```python
from build123d import *

# Parameters (mm, degrees)
BOSS_EXTRUDE1_DEPTH = 65
SKETCH2_W           = 5.2
SKETCH2_H           = 2.4
CUT_EXTRUDE1_DEPTH  = 6
LPATTERN1_COUNT     = 3
LPATTERN1_PITCH     = 20
SKETCH3_W           = 12
SKETCH3_H           = 2.4
CUT_EXTRUDE2_DEPTH  = 6
FILLET1_R           = 4
FILLET2_R           = 4
SKETCH5_W           = 13.2
SKETCH5_H           = 3.1
CUT_EXTRUDE3_DEPTH  = 10
LPATTERN2_COUNT     = 2
LPATTERN2_PITCH     = 20


with BuildPart() as part:
    # Sketch1 → Boss-Extrude1 (new body)
    with BuildSketch(Plane.XY):
        Polygon((0, 0), (3.2, 0), (4.2, 0.663324958), (4.2, 3.063324958), (-1, 3.063324958), (-1, 0.663324958), align=None)
    extrude(amount=BOSS_EXTRUDE1_DEPTH)

    # Sketch2 → Cut-Extrude1 (cut)
    with BuildSketch(Plane.ZY.offset(1)):
        with Locations((3.8, 1.863324958)):
            Rectangle(SKETCH2_W, SKETCH2_H)
    cut_extrude1 = extrude(amount=-CUT_EXTRUDE1_DEPTH, mode=Mode.SUBTRACT)

    # LPattern1: Cut-Extrude1 ×3
    with Locations(*[(0, 0, i * LPATTERN1_PITCH) for i in range(1, LPATTERN1_COUNT)]):
        add(cut_extrude1, mode=Mode.SUBTRACT)

    # Sketch3 → Cut-Extrude2 (cut)
    with BuildSketch(Plane.ZY.offset(1)):
        with Locations((57.4, 1.863324958)):
            Rectangle(SKETCH3_W, SKETCH3_H)
    extrude(amount=-CUT_EXTRUDE2_DEPTH, mode=Mode.SUBTRACT)

    # Fillet1
    # the kernel refuses this fillet: 4 mm, written as the material it adds along each edge
    with BuildSketch(Plane(origin=(-1, 0.663324958, 51.4), x_dir=(0, 0, 1), z_dir=(1, 0, 0))) as fillet1_piece_1_section:
        with BuildLine():
            CenterArc((3.666060556, -4), FILLET1_R, 90, 66.421821522)
            Line((0, -2.4), (-0.073321211, -2.368))
            ThreePointArc((-0.073321211, -2.368), (-0.08, -1.2), (-0.08, 0))
            Line((-0.08, 0), (0, 0.08))
            Line((0, 0.08), (3.666060556, 0.08))
            Line((3.666060556, 0.08), (3.666060556, 0))
        make_face()
    fillet1_piece_1 = extrude(amount=5.2, mode=Mode.PRIVATE)
    fillet1_piece_1 = split(fillet1_piece_1, bisect_by=Plane(origin=(0.518931728, -0.344220367, 52.290586237), z_dir=(0.5527707983925672, 0.833333333333333, 0)), keep=Keep.TOP, mode=Mode.PRIVATE)
    fillet1_piece_1 = split(fillet1_piece_1, bisect_by=Plane(origin=(2.681068272, -0.344220367, 52.290586237), z_dir=(-0.5527707983925666, 0.8333333333333335, 0)), keep=Keep.TOP, mode=Mode.PRIVATE)
    add(fillet1_piece_1)

    # Fillet2
    # the kernel refuses this fillet: 4 mm, written as the material it adds along each edge
    with BuildSketch(Plane(origin=(-1, 0.663324958, 63.4), x_dir=(0, 1, 0), z_dir=(1, 0, 0))) as fillet2_piece_1_section:
        with BuildLine():
            CenterArc((4, -3.666060556), FILLET2_R, 113.578178478, 66.421821522)
            Line((0, -3.666060556), (-0.08, -3.666060556))
            Line((-0.08, -3.666060556), (-0.08, 0))
            Line((-0.08, 0), (0, 0.08))
            ThreePointArc((0, 0.08), (1.2, 0.08), (2.368, 0.073321211))
            Line((2.368, 0.073321211), (2.4, 0))
        make_face()
    fillet2_piece_1 = extrude(amount=5.2, mode=Mode.PRIVATE)
    fillet2_piece_1 = split(fillet2_piece_1, bisect_by=Plane(origin=(2.681068272, -0.344220367, 62.509413763), z_dir=(-0.5527707983925666, 0.8333333333333335, 0)), keep=Keep.TOP, mode=Mode.PRIVATE)
    fillet2_piece_1 = split(fillet2_piece_1, bisect_by=Plane(origin=(0.518931728, -0.344220367, 62.509413763), z_dir=(0.5527707983925672, 0.833333333333333, 0)), keep=Keep.TOP, mode=Mode.PRIVATE)
    add(fillet2_piece_1)

    # Sketch5 → Cut-Extrude3 (cut)
    with BuildSketch(Plane.ZY.offset(1)):
        with Locations((13.8, 1.113324958)):
            Rectangle(SKETCH5_W, SKETCH5_H)
    cut_extrude3 = extrude(amount=-CUT_EXTRUDE3_DEPTH, mode=Mode.SUBTRACT)

    # LPattern2: Cut-Extrude3 ×2
    with Locations(*[(0, 0, i * LPATTERN2_PITCH) for i in range(1, LPATTERN2_COUNT)]):
        add(cut_extrude3, mode=Mode.SUBTRACT)


solid = part.part
```
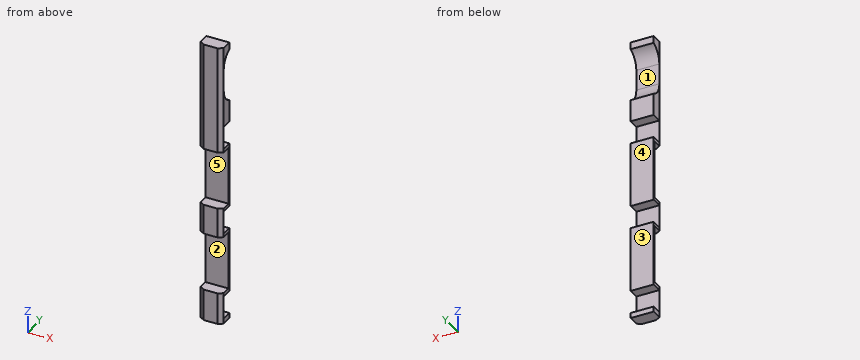
Can you work these out from the model? Positions are in its coordinate system, mm. Face numbers are marked on the shaded views. A direction names the side the tool comes from. Give positions to 0.01 mm unless a question says otherwise; leave off trailing zeros. Loops run counter-clockwise (first coordinate to the right, second up) from the corner with the lowest first, then second, coordinate; pieces in that order, holes last. Notation, with made-up numbers: M 88,-8.5 L 138,-8.5 A4 cw 138,-4.5 Z; hole C 21,-11 d9. An arc over 180 degrees is marked long. Use CSV: the item, a comma, the result in double quotes. Start each with the question number.
1. Imagine slicing it at C-C, the plane z = 50. Write out the boundary of the cut face in (x, y), plus the area to 3 significant figures.
2. If we mould it in two halves opening along Z, with no side actions, what happens to the marked faces 4 and 5? For each: released by +Z, released by -Z, zero draft, split by the parting line, or undercut.
3. If I drill on L1, parallel to Z at x = 2.45, y = 0.6; L2, parallel to Z at x = 3.95, y = 2.7; L3, parallel to Y at x = 3.7, z = 36.5, over which ranges is the centre line in solid material (lowest first)?
4. Imagine slicing it at A-A, the plane y = 1.3. Write out the boundary of the cut face in (x, z).
5. On a 3-axis mill with a long thin cutter (end or side, diameter ignored), from which of +Z, -Z, +X, -X, +Y, -Y can I reach the whole of each face in a straight line? I mean the marked faces 1, 2 and 3. Say none if no direction works.
6. For P1, Ø2.5, axis at x = 1, z = 23.5, coming from the +Y side; P2, Ø1, axis at x = 2, z = 28, coming from the -Y side, each with a flat end and sliding along its axis, tell me the tip position at first contact or that it passes through.
7. Imagine slicing it at D-D, the plane z = 8. Write out the boundary of the cut face in (x, y).
8. Imagine slicing it at B-B, the plane x = 1.5. Write out the boundary of the cut face in (y, z).
Response values:
1,outline,"M -1,0.66 L 0,0 L 3.2,0 L 4.2,0.66 L 4.2,3.06 L -1,3.06 Z"
1,area,"15.3 mm^2"
2,face 4,"zero draft"
2,face 5,"undercut"
3,L1,"0 to 7.2, 20.4 to 27.2, 40.4 to 65"
3,L2,"0 to 1.2, 6.4 to 21.2, 26.4 to 41.2, 46.4 to 51.58, 63.22 to 65"
3,L3,"2.66 to 3.06"
4,outline,"M -1,0 L 4.2,0 L 4.2,1.2 L -1,1.2 Z; M -1,6.4 L 4.2,6.4 L 4.2,7.2 L -1,7.2 Z; M -1,20.4 L 4.2,20.4 L 4.2,21.2 L -1,21.2 Z; M -1,26.4 L 4.2,26.4 L 4.2,27.2 L -1,27.2 Z; M -1,40.4 L 4.2,40.4 L 4.2,41.2 L -1,41.2 Z; M -1,46.4 L 4.2,46.4 L 4.2,52.9 L -1,52.9 Z; M -1,61.9 L 4.2,61.9 L 4.2,65 L -1,65 Z"
5,face 1,"+X, -X, +Y"
5,face 2,"+X, -X, -Y"
5,face 3,"+Z, -Z, +X, -X, +Y"
6,P1,"y = 0.66"
6,P2,"y = 2.66"
7,outline,"M -1,2.66 L 4.2,2.66 L 4.2,3.06 L -1,3.06 Z"
8,outline,"M 0,0 L 3.06,0 L 3.06,1.2 L 0.66,1.2 L 0.66,6.4 L 3.06,6.4 L 3.06,21.2 L 0.66,21.2 L 0.66,26.4 L 3.06,26.4 L 3.06,41.2 L 0.66,41.2 L 0.66,46.4 L 3.06,46.4 L 3.06,51.4 A4 cw 0.66,55.07 L 0.66,59.73 A4 cw 3.06,63.4 L 3.06,65 L 0,65 L 0,40.4 L 2.66,40.4 L 2.66,27.2 L 0,27.2 L 0,20.4 L 2.66,20.4 L 2.66,7.2 L 0,7.2 Z"
